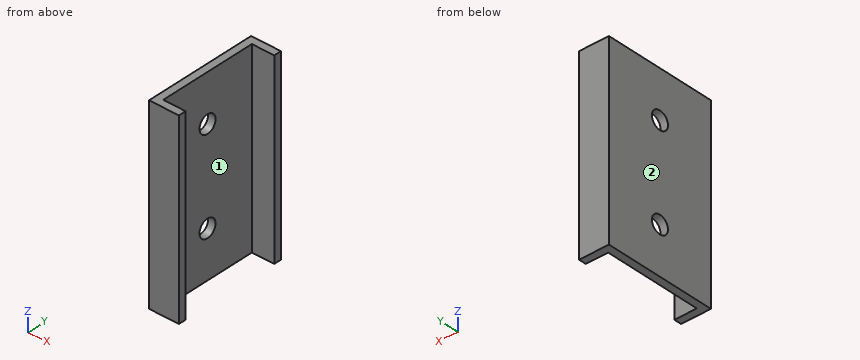
from build123d import *

# Parameters (mm, degrees)
BOSS_EXTRUDE1_DEPTH   = 20
F_6_CLEARANCE_HOLE1_D = 3.7973


with BuildPart() as part:
    # Sketch1 → Boss-Extrude1 (new body)
    with BuildSketch(Plane.XY):
        Polygon((0, 0), (6.35, 0), (6.35, 1.5875), (1.5875, 1.5875), (1.5875, 22.5875), (6.35, 22.5875), (6.35, 24.175), (0, 24.175), align=None)
    boss_extrude1 = extrude(amount=BOSS_EXTRUDE1_DEPTH)

    # #6 Clearance Hole1 (through all)
    with Locations(Plane.ZY):
        with Locations((10, 12.0875)):
            f_6_clearance_hole1 = Hole(F_6_CLEARANCE_HOLE1_D / 2)

    # Mirror1: Boss-Extrude1, #6 Clearance Hole1 across plane
    add(boss_extrude1.mirror(Plane(origin=(0, 0, 0), x_dir=(1, 0, 0), z_dir=(0, 0, -1))))
    add(f_6_clearance_hole1.mirror(Plane(origin=(0, 0, 0), x_dir=(1, 0, 0), z_dir=(0, 0, -1))), mode=Mode.SUBTRACT)


solid = part.part
Build history of the part. All positions in model axes, mm. Face numbers are marked on the shaded views. A direction names the side the tool comes from. Coordinates: 2 decimals unless noted, no trailing zeros. Write each loop counter-clockwise with the first axis right and the second up, starting at its lowest first coordinate (ties: lowest second). Pieces come first, ordered by that corner, then holes.
(1) Cut at B-B on x = 3.5. List the corners of the cut face in (y, z) (1 decimal), and give its area (3 significant figures).
(2) 3-axis set-ups, long thin cutter, end or side, ignore diameter. For the marked faces 1 and 2: which of +Z, -Z, +X, -X, +Y, -Y reach the whole face in a straight line?
(3) Pin check, flat tips, straight feed: pin 1 Ø1.5 at (y, z) = (11, 9) entering from +X; pin 2 Ø6 at (y, z) = (12.09, 10) entering from -X. Stop position of each tip, or through.
(4) Cut at C-C on x = 0.5. List the corners of the cut face in (y, z) (1 decimal), and give its area (3 significant figures).
(5) Drill centre lines: line 1 (Z direction, x = 0.75, y = 12); line 2 (Y direction, x = 0.6, z = -10) (3 decimals); line 3 (Y direction, x = 5.5, z = 11) (1 decimal). Where is each one in solid material? Low to high.
Working result:
1. outline: (0, -20) - (1.6, -20) - (1.6, 20) - (0, 20) - close; (22.6, -20) - (24.2, -20) - (24.2, 20) - (22.6, 20) - close
1. area: 127 mm2
2. face 1: +Z, -Z, +X
2. face 2: +Z, -Z, -X, +Y, -Y
3. pin 1: stops at x = 1.59
3. pin 2: stops at x = 0
4. outline: (0, -20) - (24.2, -20) - (24.2, 20) - (0, 20) - close; hole circle Ø3.8 at (12.1, -10); hole circle Ø3.8 at (12.1, 10)
4. area: 944 mm2
5. line 1: z = -20 to -11.9, -8.1 to 8.1, 11.9 to 20
5. line 2: y = 0 to 10.189, 13.986 to 24.175
5. line 3: y = 0 to 1.6, 22.6 to 24.2
